For this review, take the finished solid that the model builds, in its own axes (mm). A direction names the side the tool comes from. Coordinates: 2 decimals unless noted, no trailing zeros. Loops run counter-clockwise (first coordinate to the right, second up) from the corner with the lowest first, then second, coordinate; pieces in that order, holes last. Notation, with made-up numbers: M 52,76.5 L 63,76.5 A19 cw 63,96.5 Z; hole C -15,50 d7. An arc over 180 degrees is marked long. Write item = value, one per line.
from build123d import *

# Parameters (mm, degrees)
EXTRUDE_1_DEPTH          = 6
EXTRUDE_2_DEPTH          = 50
EXTRUDE_3_REACH          = 116.36
EXTRUDE_4_REACH          = 109.318
PATTERN_CIRCULAR_1_COUNT = 5
CUT_EXTRUDE_START        = 34.260416
CUT_EXTRUDE_2_DEPTH      = 15.739584
SHELL_2_T                = 4
CUT_EXTRUDE_3_DEPTH      = 4
PATTERN_CIRCULAR_2_COUNT = 5
MIRROR_2_COPY_1_DEPTH    = 4
MIRROR_2_COPY_2_DEPTH    = 4
MIRROR_2_COPY_3_DEPTH    = 4
MIRROR_2_COPY_4_DEPTH    = 4


with BuildPart() as part:
    # 草图1 → 凸台-拉伸1 (new body)
    with BuildSketch(Plane(origin=(0, 0, 0), x_dir=(1, 0, 0), z_dir=(0, 1, 0))):
        Polygon((6, 63.6928095), (-6, 63.6928095), (-58.72135955, 25.388499653), (-62.429563482, 13.975821457), (-42.291796068, -48.001853791), (-32.583592135, -55.055276819), (32.583592135, -55.055276819), (42.291796068, -48.001853791), (62.429563482, 13.975821457), (58.72135955, 25.388499653), align=None)
    extrude(amount=EXTRUDE_1_DEPTH)

    # 草图2 → 凸台-拉伸2 (add)
    with BuildSketch(Plane(origin=(0, 6, 0), x_dir=(1, 0, 0), z_dir=(0, 1, 0))):
        Polygon((-6, 8.258291523), (-9.708203932, -3.154386673), (0, -10.2078097), (9.708203932, -3.154386673), (6, 8.258291523), align=None)
    extrude(amount=EXTRUDE_2_DEPTH)

    # 草图3 → 凸台-拉伸3 (add, up to next)
    with BuildSketch(Plane(origin=(22.048945114, 30.347769421, 7.164136549), x_dir=(-0.8164965809277247, 0.5619055660577269, 0.1326479105251229), z_dir=(-0.5773502691896276, -0.7946544722917646, -0.18759247408508062)), mode=Mode.PRIVATE) as extrude_3_sk1:
        Polygon((-49.45595525, 14.980471634), (-24.792327887, -45.339238172), (15.114259472, 6.179944577), align=None)
    extrude_3_tool1 = extrude(extrude_3_sk1.sketch, amount=EXTRUDE_3_REACH, mode=Mode.PRIVATE) - part.part
    extrude_3 = extrude_3_tool1.solids().sort_by_distance((38.143188, 17.420139, 12.393473))[0]
    add(extrude_3)

    # 草图5 → 凸台-拉伸4 (add, up to next)
    with BuildSketch(Plane(origin=(19.294598211, 32.825931131, -6.26919499), x_dir=(0.8660254037844378, -0.49112347318842436, 0.09379623704254153), z_dir=(0.5000000000000017, 0.8506508083520388, -0.16245984811645525)), mode=Mode.PRIVATE) as extrude_4_sk1:
        Polygon((-11.069414635, -10.650937771), (49.807967622, 12.602153105), (45.526102544, 23.812221413), (-15.351279712, 0.559130537), align=None)
    extrude_4_tool1 = extrude(extrude_4_sk1.sketch, amount=-EXTRUDE_4_REACH, mode=Mode.PRIVATE) - part.part
    extrude_4 = extrude_4_tool1.solids().sort_by_distance((34.214782, 23.130208, -11.117056))[0]
    add(extrude_4)

    # 阵列(圆周)1: 凸台-拉伸3, 凸台-拉伸4 ×5 about axis
    pattern_circular_1_axis = Axis((0, 0, 0), (0, 1, 0))
    add([extrude_3.rotate(pattern_circular_1_axis, i * 360 / PATTERN_CIRCULAR_1_COUNT) for i in range(1, PATTERN_CIRCULAR_1_COUNT)])
    add([extrude_4.rotate(pattern_circular_1_axis, i * 360 / PATTERN_CIRCULAR_1_COUNT) for i in range(1, PATTERN_CIRCULAR_1_COUNT)])

    # 草图2<2> → 切除-拉伸2 (cut)
    with BuildSketch(Plane(origin=(0, 6, 0), x_dir=(1, 0, 0), z_dir=(0, 1, 0)).offset(CUT_EXTRUDE_START)):
        Polygon((-6, 8.258291523), (-9.708203932, -3.154386673), (0, -10.2078097), (9.708203932, -3.154386673), (6, 8.258291523), align=None)
    extrude(amount=CUT_EXTRUDE_2_DEPTH, mode=Mode.SUBTRACT)

    # 镜向1: part across plane


with BuildPart() as part_1:
    add(part.part)
    add(part.part.mirror(Plane.ZX))

    # 抽壳2 (no face opened: a closed hollow body)
    add(offset(amount=-SHELL_2_T, mode=Mode.PRIVATE), mode=Mode.SUBTRACT)

    # 草图6 → 切除-拉伸3 (cut)
    with BuildSketch(Plane(origin=(22.048945114, 30.347769421, 7.164136549), x_dir=(0.8164965809277248, -0.5619055660577268, -0.13264791052512276), z_dir=(0.5773502691896275, 0.7946544722917647, 0.18759247408508056))):
        Polygon((-11.411800298, 4.66607666), (24.252146374, -41.375880513), (46.29367759, 12.530981891), align=None)
    cut_extrude_3 = extrude(amount=-CUT_EXTRUDE_3_DEPTH, mode=Mode.SUBTRACT)

    # 阵列(圆周)2: 切除-拉伸3 ×5 about axis
    pattern_circular_2_axis = Axis((0, 0, 0), (0, 1, 0))
    for i in range(1, PATTERN_CIRCULAR_2_COUNT):
        add(cut_extrude_3.rotate(pattern_circular_2_axis, i * 360 / PATTERN_CIRCULAR_2_COUNT), mode=Mode.SUBTRACT)

    # 镜向2: 切除-拉伸3 across plane
    add(cut_extrude_3.mirror(Plane.ZX), mode=Mode.SUBTRACT)

    # 镜向2 copy 1 sketch → 镜向2 copy 1 (cut)
    with BuildSketch(Plane(origin=(13.626997497, -30.347769421, -18.755952985), x_dir=(0.12615565967785208, 0.5619055660577268, -0.8175248524446163), z_dir=(0.3568220897730911, -0.7946544722917647, -0.4911234731884244))):
        Polygon((-11.411800298, -4.66607666), (24.252146374, 41.375880513), (46.29367759, -12.530981891), align=None)
    extrude(amount=-MIRROR_2_COPY_1_DEPTH, mode=Mode.SUBTRACT)

    # 镜向2 copy 2 sketch → 镜向2 copy 2 (cut)
    with BuildSketch(Plane(origin=(-13.626997497, -30.347769421, -18.755952985), x_dir=(-0.7385280953736475, 0.5619055660577268, -0.37261023493339274), z_dir=(-0.3568220897730909, -0.7946544722917647, -0.49112347318842464))):
        Polygon((-11.411800298, -4.66607666), (24.252146374, 41.375880513), (46.29367759, -12.530981891), align=None)
    extrude(amount=-MIRROR_2_COPY_2_DEPTH, mode=Mode.SUBTRACT)

    # 镜向2 copy 3 sketch → 镜向2 copy 3 (cut)
    with BuildSketch(Plane(origin=(-22.048945114, -30.347769421, 7.164136549), x_dir=(-0.5825911242654904, 0.5619055660577267, 0.5872390626996962), z_dir=(-0.5773502691896276, -0.7946544722917646, 0.18759247408508029))):
        Polygon((-11.411800298, -4.66607666), (24.252146374, 41.375880513), (46.29367759, -12.530981891), align=None)
    extrude(amount=-MIRROR_2_COPY_3_DEPTH, mode=Mode.SUBTRACT)

    # 镜向2 copy 4 sketch → 镜向2 copy 4 (cut)
    with BuildSketch(Plane(origin=(0, -30.347769421, 23.183632872), x_dir=(0.37846697903356086, 0.5619055660577268, 0.7355439352034356), z_dir=(0, -0.7946544722917647, 0.6070619982066882))):
        Polygon((-11.411800298, -4.66607666), (24.252146374, 41.375880513), (46.29367759, -12.530981891), align=None)
    extrude(amount=-MIRROR_2_COPY_4_DEPTH, mode=Mode.SUBTRACT)


solid = part_1.part
Q1. Draft analysis for pull direction Z (two halves, no side actions). For faces 1 (the face through (-56.75, 0.05, -18.51)), 2 (the face through (34.083, -22.95, -12.464)), 3 (the face through (0, 40.26, 1)), state which applies: +Z half, -Z half, draft (parallel to the pull), parting line (faces both ways), or undercut.
Solved:
face_1 = undercut
face_2 = -Z half
face_3 = draft
Q2. Add section B-B (z = -31). State how many separate pieces and enclosed holes the cut face has, and give its area (3 significant figures).
Solved:
separate_pieces = 4
enclosed_holes = 0
area = 301 mm²
Q3. For line 1 along Y through (x, z) = (34.5, 48.5); line 2 along Z through (x, y) = (10, -2.5); line 3 along Y through (x, z) = (-28.5, 40.5), list the stretches that pass through material, from the lowest coordinate up.
Solved:
line_1 = -8.58 to -3.88, 3.88 to 8.58
line_2 = -60.79 to -55.84, 51.06 to 55.06
line_3 = -14.76 to -10.06, 10.06 to 14.76
Q4. Machinability: for faces 4 (the face through (0, -36.26, 1)), 5 (the face through (22.39, -22.95, 28.56)), which of the approach directions +Z, -Z, +X, -X, +Y, -Y give a long, thin tool a straight path to every point of the face, cutting with its end or side? Answer none if there is none.
Solved:
face_4 = none
face_5 = +Z, +X, -Y
Q5. For pin 1 Ø1 at (x, y) = (25.5, 5.5) entering from -Z; pin 2 Ø1 at (x, y) = (-6, 27.5) entering from +Z; pin 3 Ø12 at (y, z) = (-23.5, -16.5) entering from +X, all flat-tipped, find the tip position at first contact; note any pin that passes through.
Solved:
pin_1 = -49.89
pin_2 = -19.87
pin_3 = 42.23
Q6. Add section A-A (y = 0.5). Write out the cut boundary in (x, z).
Solved:
outline = M -62.43,-13.98 L -58.72,-25.39 L -6,-63.69 L 6,-63.69 L 58.72,-25.39 L 62.43,-13.98 L 42.29,48 L 32.58,55.06 L -32.58,55.06 L -42.29,48 Z; hole M -58.22,-13.98 L -55.32,-22.92 L -4.7,-59.69 L 4.7,-59.69 L 55.32,-22.92 L 58.22,-13.98 L 38.89,45.53 L 31.28,51.06 L -31.28,51.06 L -38.89,45.53 Z
